```python
from build123d import *

# Parameters (mm, degrees)
F1_DEPTH = 0.79375
F2_R     = 0.635
F3_R     = 5.08


with BuildPart() as f1:
    # F0 (on Front) → F1 (new body, symmetric)
    with BuildSketch(Plane.XZ):
        with BuildLine():
            Line((-5.08, -9.4615), (5.08, -9.4615))
            Line((5.08, -9.4615), (5.08, 9.4615))
            Line((5.08, 9.4615), (-5.08, 9.4615))
            add(Edge.make_bspline(
                [(-5.08, 9.4615), (-5.08, 6.1859851204), (-14.0601360435, 7.136818114), (-16.564456746, 2.7273960877), (-17.78, 0.79375)],
                knots=[0, 0, 0, 0, 0.5228302589, 1, 1, 1, 1], degree=3))
            Line((-17.78, 0.79375), (-5.08, 0.79375))
            Line((-5.08, 0.79375), (-5.08, -0.79375))
            Line((-5.08, -0.79375), (-17.78, -0.79375))
            add(Edge.make_bspline(
                [(-5.08, -9.4615), (-5.08, -6.1859851204), (-14.0601360435, -7.136818114), (-16.564456746, -2.7273960877), (-17.78, -0.79375)],
                knots=[0, 0, 0, 0, 0.5228302589, 1, 1, 1, 1], degree=3))
        make_face()
    extrude(amount=F1_DEPTH, both=True)

    # F2
    f2_edges = [f1.edges().sort_by_distance(p)[0] for p in [
        (5.08, 0, 9.4615),
        (5.08, 0, -9.4615),
    ]]
    fillet(f2_edges, radius=F2_R)

    # F3
    f3_edges = [f1.edges().sort_by_distance(p)[0] for p in [
        (-5.08, 0.396875, 9.4615),
        (-5.08, -0.396875, 9.4615),
        (-5.08, 0.396875, -9.4615),
        (-5.08, -0.396875, -9.4615),
    ]]
    fillet(f3_edges, radius=F3_R)


solid = f1.part
```
Could you check a few things on this model? Use its own coordinates, in mm. A direction names the side the tool comes from. Round coordinates to 2 decimals unless told otherwise and drop trailing zeros. Write each question's results on one line, items separated by ' | '. Start each with the question number.
1. I'm going to push a flat-ended pin straight in: pin 1 Ø0.5 at (x, y) = (-10.5, 0) entering from -Z. Where does the tip first touch, or does it pass through?
2. On a 3-axis mill with a long thin cutter (end or side, diameter ignored), from which of +Z, -Z, +X, -X, +Y, -Y can I reach the whole of each face in a straight line? I mean faces 4 (the face through (-4, 0.794, 0)), 5 (the face through (-12, 0, 0.794)). Say none if no direction works.
3. Thinking about a two-plate mould opening in Z: for faces 1 (the face through (-5.08, 0, 0)), 2 (the face through (1, 0, -9.462)), 3 (the face through (5.08, 0, 0)), which applies, +Z half, -Z half, draft (parallel to the pull), parting line (faces both ways), or undercut?
4. I need wall thicknesses on L1, parallel to Z at x = -13.25, y = 0.3; L2, parallel to Z at x = -6.25, y = 0.1; L3, parallel to X at y = 0.1, z = -0.5. Which ranges of each line are inside material? Lowest first, please. Write a range as from..to.
Result sheet:
1) pin 1: stops at z = -6.25
2) face 4: +Z, -Z, +X, -X, +Y | face 5: -X, +Y, -Y
3) face 1: undercut | face 2: -Z half | face 3: draft
4) L1: z = -5.51..-0.79, 0.79..5.51 | L2: z = -7.34..-0.79, 0.79..7.34 | L3: x = -5.08..5.08
